Input: part model. Units: mm. Frame: model coordinates. A direction names the side the tool comes from. Give positions to 0.01 mm unless a question says otherwise; leave off trailing zeros. Write each loop counter-clockwise with the first axis right and the second up, starting at its lowest first coordinate (ties: lowest second). Pieces come first, ordered by that corner, then holes.
```python
from build123d import *


with BuildPart() as part:
    # Sketch1 → Revolve1 (revolve)
    with BuildSketch(Plane(origin=(0, 0, 0), x_dir=(-1, 0, 0), z_dir=(0, 0, -1))):
        with BuildLine():
            Line((-5.925, -4.5), (-5.925, -3.669134295))
            ThreePointArc((-5.925, -3.669134295), (-6.6, -2.5), (-5.925, -1.330865705))
            Line((-5.925, -1.330865705), (-5.925, -0.5))
            Line((-5.925, -0.5), (-6.0435, -0.5))
            Line((-6.0435, -0.5), (-6.0435, -0.49))
            Line((-6.0435, -0.49), (-4.4935, -0.49))
            Line((-4.4935, -0.49), (-4.4935, 0))
            Line((-4.4935, 0), (-5.8035, 0))
            Line((-5.8035, 0), (-6.0435, -0.24))
            Line((-6.0435, -0.24), (-6.0435, 0))
            Line((-6.0435, 0), (-7.3, 0))
            ThreePointArc((-7.3, 0), (-7.441421356, -0.058578644), (-7.5, -0.2))
            Line((-7.5, -0.2), (-7.5, -4.8))
            ThreePointArc((-7.5, -4.8), (-7.441421356, -4.941421356), (-7.3, -5))
            Line((-7.3, -5), (-6.0435, -5))
            Line((-6.0435, -5), (-6.0435, -4.76))
            Line((-6.0435, -4.76), (-5.8035, -5))
            Line((-5.8035, -5), (-4.4935, -5))
            Line((-4.4935, -5), (-4.4935, -4.51))
            Line((-4.4935, -4.51), (-6.0435, -4.51))
            Line((-6.0435, -4.51), (-6.0435, -4.5))
            Line((-6.0435, -4.5), (-5.925, -4.5))
        make_face()
    revolve(axis=Axis((0, -5.001250002, 0), (0, 1, 0)))


solid = part.part
```
Item 1: Mould query, pull axis X, two halves, no side actions, for faces 1 (the flat face through (-4.4, -5, -4.4)), 2 (the cylindrical face through (-7.493, -2.532, -0.33)), 3 (the cylindrical face through (5.65, -4.08, -1.78)). Classes: +X half, -X half, draft (parallel to the pull), parting line (faces both ways), or undercut.
Item 2: Section B-B (y = -2.85). Return loops of the section in (x, z).
Item 3: Set-up query: faces 4 (the flat face through (0, -4.51, -5)), 5 (the flat face through (4.4, 0, -4.4)). Return all of +Z, -Z, +X, -X, +Y, -Y with unobstructed straight access to the full face (end or side cutting, diameter ignored); none if empty.
Item 4: Section A-A (y = -1). Return loops of the section in (x, z) (3 decimals), and give its area (3 significant figures).
Item 5: Ray query, line 1 (Y direction, x = 4.5, z = 2.5); line 2 (X direction, y = -0.65, z = 0) (3 decimals); line 3 (X direction, y = -0.4, z = 0). Return the intervals inside material, ascending.
Solved:
1. face 1: draft
1. face 2: parting line
1. face 3: undercut
2. outline: circle Ø15 at (0, 0); hole circle Ø13.11 at (0, 0)
3. face 4: none
3. face 5: +Z, -Z, +X, -X, +Y
4. outline: circle Ø15 at (0, 0); hole circle Ø11.85 at (0, 0)
4. area: 66.4 mm2
5. line 1: y = -5 to -4.51, -0.49 to 0
5. line 2: x = -7.5 to -5.925, 5.925 to 7.5
5. line 3: x = -7.5 to -4.49, 4.49 to 7.5
